```python
from build123d import *

# Parameters (mm, degrees)
SKETCH2_R               = 13
SKETCH2_R_2             = 7.5
BOSS_EXTRUDE2_DEPTH     = 10
CUT_EXTRUDE1_DEPTH      = 105.791459576
CUT_EXTRUDE1_DEPTH_BACK = 105.791459576
SKETCH5_R               = 1.83
SKETCH5_R_2             = 3.05
CUT_EXTRUDE2_DEPTH      = 106.770979007
HUB_CUTOUT_DEPTH        = 7
SKETCH8_R               = 6.5
CUT_EXTRUDE4_DEPTH      = 3
CUT_EXTRUDE5_DEPTH      = 105.791459576
CUT_EXTRUDE5_DEPTH_BACK = 105.791459576
SKETCH9_R               = 1.55
CUT_EXTRUDE6_DEPTH      = 5.5
FILLET1_R               = 2
CUT_EXTRUDE7_START      = 2.5
CUT_EXTRUDE7_DEPTH      = 103.291459576
FILLET2_R               = 2
FILLET2_OF_MIRROR1_R    = 2
SKETCH12_R              = 4
SKETCH12_R_2            = 1.55
BOSS_EXTRUDE3_DEPTH     = 4
FILLET3_START           = -14
FILLET3_2_DEPTH         = 4
BOSS_EXTRUDE4_START     = 5.5
SKETCH13_R              = 2.5
SKETCH13_R_2            = 1.5
BOSS_EXTRUDE4_DEPTH     = 0.5
BOSS_EXTRUDE5_START     = -5
SKETCH13_2_R            = 2.5
SKETCH13_2_R_2          = 1.5
BOSS_EXTRUDE5_DEPTH     = 0.5
FILLET4_R               = 5
SKETCH15_R              = 4
CUT_EXTRUDE8_DEPTH      = 3


with BuildPart() as part:
    # Sketch2 → Boss-Extrude2 (new, symmetric)
    with BuildSketch(Plane.XY):
        Circle(SKETCH2_R)
        with BuildLine():
            Line((70, 7.5), (1.025771359, 12.959467316))
            ThreePointArc((1.025771359, 12.959467316), (9.548168088, 8.822272166), (13, 0))
            ThreePointArc((13, 0), (9.548168088, -8.822272166), (1.025771359, -12.959467316))
            Line((1.025771359, -12.959467316), (70, -7.5))
            Line((70, -7.5), (70, 7.5))
        make_face()
        with BuildLine():
            Line((96, 7.5), (70, 7.5))
            Line((70, 7.5), (70, -7.5))
            Line((70, -7.5), (96, -7.5))
            ThreePointArc((96, -7.5), (88.5, 0), (96, 7.5))
        make_face()
        with Locations((96, 0)):
            Circle(SKETCH2_R_2)
        Circle(SKETCH2_R)
    extrude(amount=BOSS_EXTRUDE2_DEPTH, both=True)

    # Sketch4 → Cut-Extrude1 (cut, two sides: drawn at the far end of the back side and taken through both)
    with BuildSketch(Plane(origin=(0, 0, 0), x_dir=(1, 0, 0), z_dir=(0, 1, 0)).offset(-CUT_EXTRUDE1_DEPTH_BACK)):
        Polygon((-13, 7.5), (50, 7.5), (80, 10), (-13, 10), align=None)
        Polygon((-13, -7.5), (50, -7.5), (80, -10), (-13, -10), align=None)
    extrude(amount=CUT_EXTRUDE1_DEPTH + CUT_EXTRUDE1_DEPTH_BACK, mode=Mode.SUBTRACT)

    # Sketch5 → Cut-Extrude2 (cut, through all)
    with BuildSketch(Plane.XY.offset(7.5)):
        with Locations((-6.914797213, 6.914797213)):
            Circle(SKETCH5_R)
        with Locations((6.914797213, 6.914797213)):
            Circle(SKETCH5_R)
        with Locations((6.914797213, -6.914797213)):
            Circle(SKETCH5_R)
        with Locations((-6.914797213, -6.914797213)):
            Circle(SKETCH5_R)
        Circle(SKETCH5_R_2)
    extrude(amount=-CUT_EXTRUDE2_DEPTH, mode=Mode.SUBTRACT)

    # Sketch7 → hub cutout (cut)
    with BuildSketch(Plane.XY.offset(7.5)):
        with BuildLine():
            ThreePointArc((-7.281143007, 10.769631215), (-13, 0), (-7.281143007, -10.769631215))
            ThreePointArc((-7.281143007, -10.769631215), (-6.15529138, -10.711783559), (-5.093815501, -10.332103173))
            ThreePointArc((-5.093815501, -10.332103173), (-4.17580433, -10.057753531), (-3.223255475, -10.161014917))
            ThreePointArc((-3.223255475, -10.161014917), (0, -10.66), (3.223255475, -10.161014917))
            ThreePointArc((3.223255475, -10.161014917), (4.17580433, -10.057753531), (5.093815501, -10.332103173))
            ThreePointArc((5.093815501, -10.332103173), (9.652858062, -9.652858062), (10.332103173, -5.093815501))
            ThreePointArc((10.332103173, -5.093815501), (10.057753531, -4.17580433), (10.161014917, -3.223255475))
            ThreePointArc((10.161014917, -3.223255475), (10.66, 0), (10.161014917, 3.223255475))
            ThreePointArc((10.161014917, 3.223255475), (10.057753531, 4.17580433), (10.332103173, 5.093815501))
            ThreePointArc((10.332103173, 5.093815501), (9.652858062, 9.652858062), (5.093815501, 10.332103173))
            ThreePointArc((5.093815501, 10.332103173), (4.17580433, 10.057753531), (3.223255475, 10.161014917))
            ThreePointArc((3.223255475, 10.161014917), (0, 10.66), (-3.223255475, 10.161014917))
            ThreePointArc((-3.223255475, 10.161014917), (-4.17580433, 10.057753531), (-5.093815501, 10.332103173))
            ThreePointArc((-5.093815501, 10.332103173), (-6.15529138, 10.711783559), (-7.281143007, 10.769631215))
        make_face()
    extrude(amount=-HUB_CUTOUT_DEPTH, mode=Mode.SUBTRACT)

    # Sketch8 → Cut-Extrude4 (cut)
    with BuildSketch(Plane.XY.offset(0.5)):
        Circle(SKETCH8_R)
    extrude(amount=-CUT_EXTRUDE4_DEPTH, mode=Mode.SUBTRACT)

    # Sketch9 → Cut-Extrude5 (cut, two sides: drawn at the far end of the back side and taken through both)
    with BuildSketch(Plane.XY.offset(-CUT_EXTRUDE5_DEPTH_BACK)):
        with Locations((96, 0)):
            Circle(SKETCH9_R)
    extrude(amount=CUT_EXTRUDE5_DEPTH + CUT_EXTRUDE5_DEPTH_BACK, mode=Mode.SUBTRACT)

    # Sketch10 → Cut-Extrude6 (cut, symmetric)
    with BuildSketch(Plane.XY):
        Polygon((84, 0), (62.184725581, 12.595054558), (110.068063566, 12.595054558), (110.068063566, -12.520209035), (62.31436183, -12.520209035), align=None)
    extrude(amount=CUT_EXTRUDE6_DEPTH, both=True, mode=Mode.SUBTRACT)

    # Fillet1
    fillet1_edges = [part.edges().sort_by_distance(p)[0] for p in [
        (84, 0, 0),
    ]]
    fillet(fillet1_edges, radius=FILLET1_R)

    # Sketch11 → Cut-Extrude7 (cut, through all)
    with BuildSketch(Plane.XY.offset(CUT_EXTRUDE7_START)):
        Polygon((13.951045221, 0), (20.381756661, 7.414886386), (70.904413477, 3.415903011), (70.904413477, 0), (70.904413477, -3.415903011), (20.381756661, -7.414886386), align=None)
    cut_extrude7 = extrude(amount=CUT_EXTRUDE7_DEPTH, mode=Mode.SUBTRACT)

    # Fillet2
    fillet2_edges = [part.edges().sort_by_distance(p)[0] for p in [
        (13.951045221, 0, 5),
        (20.381756661, 7.414886386, 5),
        (20.381756661, -7.414886386, 5),
        (70.904413477, -3.415903011, 5.871017228),
        (70.904413477, 3.415903011, 5.871017228),
    ]]
    fillet(fillet2_edges, radius=FILLET2_R)

    # Mirror1: Cut-Extrude7 across plane
    add(cut_extrude7.mirror(Plane.XY), mode=Mode.SUBTRACT)

    # Fillet2 of Mirror1
    fillet2_of_mirror1_edges = [part.edges().sort_by_distance(p)[0] for p in [
        (13.951045221, 0, -5),
        (20.381756661, 7.414886386, -5),
        (20.381756661, -7.414886386, -5),
        (70.904413477, -3.415903011, -5.871017228),
        (70.904413477, 3.415903011, -5.871017228),
    ]]
    fillet(fillet2_of_mirror1_edges, radius=FILLET2_OF_MIRROR1_R)

    # Sketch12 → Boss-Extrude3 (add)
    with BuildSketch(Plane(origin=(0, 0, -10), x_dir=(-1, 0, 0), z_dir=(0, 0, -1))):
        with Locations(Location((-96, 0, 0), (0, 0, 180))):
            Circle(SKETCH12_R)
        with Locations(Location((-96, 0, 0), (0, 0, 180))):
            Circle(SKETCH12_R_2, mode=Mode.SUBTRACT)
    extrude(amount=BOSS_EXTRUDE3_DEPTH)

    # Fillet3: read off the stored shape, not the designer's step
    # Fillet3 outline → Fillet3 (revolve)
    with BuildSketch(Plane(origin=(96, 0, 0), x_dir=(1, 0, 0), z_dir=(0, -1, 0))):
        with BuildLine():
            ThreePointArc((4, -14), (7.527864045, -11.05572809), (12, -10))
            Line((12, -10), (4, -10))
            Line((4, -10), (4, -14))
        make_face()
    revolve(axis=Axis((96, 0, 0), (0, 0, 1)))

    # Fillet3 2 outline → Fillet3 2 (cut)
    with BuildSketch(Plane.XY.offset(FILLET3_START)):
        with BuildLine():
            ThreePointArc((96, 7.5), (103.5, 0), (96, -7.5))
            Line((96, -7.5), (85, -7.5))
            Line((85, -7.5), (85, -13))
            Line((85, -13), (109, -13))
            Line((109, -13), (109, 13))
            Line((109, 13), (85, 13))
            Line((85, 13), (85, 7.5))
            Line((85, 7.5), (96, 7.5))
        make_face()
    extrude(amount=FILLET3_2_DEPTH, mode=Mode.SUBTRACT)

    # Sketch13 → Boss-Extrude4 (add)
    with BuildSketch(Plane.XY.offset(BOSS_EXTRUDE4_START)):
        with Locations((96, 0)):
            Circle(SKETCH13_R)
        with Locations((96, 0)):
            Circle(SKETCH13_R_2, mode=Mode.SUBTRACT)
    extrude(amount=-BOSS_EXTRUDE4_DEPTH)

    # Sketch13<2> → Boss-Extrude5 (add)
    with BuildSketch(Plane.XY.offset(BOSS_EXTRUDE5_START)):
        with Locations((96, 0)):
            Circle(SKETCH13_2_R)
        with Locations((96, 0)):
            Circle(SKETCH13_2_R_2, mode=Mode.SUBTRACT)
    extrude(amount=-BOSS_EXTRUDE5_DEPTH)

    # Fillet4
    # the kernel refuses this fillet: 5 mm, written as the material it adds along each edge
    with BuildSketch(Plane(origin=(96, 0, 5.5), x_dir=(1, 0, 0), z_dir=(0, -1, 0))) as fillet4_piece_1:
        with BuildLine():
            CenterArc((4.679449472, -5), FILLET4_R, 90, 25.841932763)
            Line((2.5, -0.5), (2.456411011, -0.41))
            ThreePointArc((2.456411011, -0.41), (2.4, -0.25), (2.4, 0))
            Line((2.4, 0), (2.5, 0.1))
            Line((2.5, 0.1), (4.679449472, 0.1))
            Line((4.679449472, 0.1), (4.679449472, 0))
        make_face()
    revolve(axis=Axis((96, 0, 5.5), (0, 0, 1)))
    with BuildSketch(Plane(origin=(96, 0, -5.5), x_dir=(1, 0, 0), z_dir=(0, -1, 0))) as fillet4_piece_2:
        with BuildLine():
            CenterArc((4.679449472, 5), FILLET4_R, 244.158067237, 25.841932763)
            Line((2.5, 0.5), (2.456411011, 0.41))
            ThreePointArc((2.456411011, 0.41), (2.4, 0.25), (2.4, 0))
            Line((2.4, 0), (2.5, -0.1))
            Line((2.5, -0.1), (4.679449472, -0.1))
            Line((4.679449472, -0.1), (4.679449472, 0))
        make_face()
    revolve(axis=Axis((96, 0, -5.5), (0, 0, 1)))

    # Sketch15 → Cut-Extrude8 (cut)
    with BuildSketch(Plane(origin=(0, 0, -7.5), x_dir=(-1, 0, 0), z_dir=(0, 0, -1))):
        with Locations((6.914797213, -6.914797213)):
            Circle(SKETCH15_R)
        with Locations((-6.914797213, -6.914797213)):
            Circle(SKETCH15_R)
        with Locations((6.914797213, 6.914797213)):
            Circle(SKETCH15_R)
        with Locations((-6.914797213, 6.914797213)):
            Circle(SKETCH15_R)
    extrude(amount=-CUT_EXTRUDE8_DEPTH, mode=Mode.SUBTRACT)


solid = part.part
```
Model file for the job. Use its own axes, mm. A direction names the side the tool comes from. Give positions to 0.01 mm unless a question says otherwise; leave off trailing zeros. Write each loop counter-clockwise with the first axis right and the second up, starting at its lowest first coordinate (ties: lowest second). Pieces come first, ordered by that corner, then holes. Notation, with made-up numbers: (-1.75, 34.5) -> (43.25, 34.5) arc R16 cw to (43.25, 55.5) -> close; hole circle Ø2 at (50.5, 24). An arc over 180 degrees is marked (long way). Use CSV: the item, a comma, the result in double quotes. Start each with the question number.
1) Tool access for faces 4 (the flat face through (96, -2, -5)), 5 (the flat face through (11, 0, -7.5)), 6 (the flat face through (-6, 5, -4.5)), 7 (the cylindrical face through (-4.19, -10.06, 4.05)): list every direction of +Z, -Z, +X, -X, +Y, -Y with a clear straight run to the whole face (end or side of a thin tool).
2) Two-plate mould, pull along X, no slides. Class faces 1 (the cylindrical face through (10.06, -4.19, 4.05)), 2 (the cylindrical face through (103.5, -0.16, 7.78)), 3 (the cylindrical face through (70.36, 2.94, 5.92)): released by +X, released by -X, zero draft, split by the parting line, or undercut.
3) Cut at D-D on x = 33. List the corners of the cut face in (y, z).
4) Cut at C-C on x = 61.5. List the corners of the cut face in (y, z), plus the area to 3 significant figures.
5) Pin check, flat tips, straight feed: P1, Ø12, axis at x = 37.5, z = 0.5, coming from the +Y side; P2, Ø9, axis at x = 8, y = -6.5, coming from the -Z side; P3, Ø5, axis at y = -8, z = 6.5, coming from the -X side; P4, Ø3.5, axis at x = 6.91, y = 6.91, coming from the -Z side. Stop position of each tip, or through.
6) Cut at A-A on x = 0. List the corners of the cut face in (y, z), plus the area to 3 significant figures.
7) Cut at B-B on y = 0. Count the separate pieces of the cut face and the enclosed holes in it, plus the area to 3 significant figures.
8) Drill centre lines: L1, parallel to X at y = 0, z = 4.5; L2, parallel to X at y = 0, z = 8.5; L3, parallel to X at y = 1, z = -2.75. Where is each one in solid material? Low to high.
Final values:
1,face 4,"+X, +Y, -Y"
1,face 5,"-Z, -X, +Y, -Y"
1,face 6,"-Z"
1,face 7,"+Z"
2,face 1,"released by -X"
2,face 2,"released by +X"
2,face 3,"undercut"
3,outline,"(-10.43, -7.5) -> (-6.42, -7.5) -> (-6.42, -2.5) -> (6.42, -2.5) -> (6.42, -7.5) -> (10.43, -7.5) -> (10.43, 7.5) -> (6.42, 7.5) -> (6.42, 2.5) -> (-6.42, 2.5) -> (-6.42, 7.5) -> (-10.43, 7.5) -> close"
4,outline,"(-8.17, -8.46) -> (-4.16, -8.46) -> (-4.16, -2.5) -> (4.16, -2.5) -> (4.16, -8.46) -> (8.17, -8.46) -> (8.17, 8.46) -> (4.16, 8.46) -> (4.16, 2.5) -> (-4.16, 2.5) -> (-4.16, 8.46) -> (-8.17, 8.46) -> close"
4,area,"177 mm2"
5,P1,"stops at y = 10.55"
5,P2,"stops at z = -7.5"
5,P3,"stops at x = -5.45"
5,P4,"passes through"
6,outline,"(-13, -7.5) -> (-3.05, -7.5) -> (-3.05, -2.5) -> (-6.5, -2.5) -> (-6.5, 0.5) -> (-10.66, 0.5) -> (-10.66, 7.5) -> (-13, 7.5) -> close; (3.05, -7.5) -> (13, -7.5) -> (13, 7.5) -> (10.66, 7.5) -> (10.66, 0.5) -> (6.5, 0.5) -> (6.5, -2.5) -> (3.05, -2.5) -> close"
6,area,"171 mm2"
7,separate pieces,"4"
7,enclosed holes,"0"
7,area,"882 mm2"
8,L1,"x = 10.66 to 14.6, 70.9 to 82"
8,L2,"x = 70.9 to 94.45, 97.55 to 103.5"
8,L3,"x = -12.96 to -2.88, 2.88 to 14.87, 70.9 to 81.73"
